from build123d import *

# Parameters (mm, degrees)
SKETCH1_R           = 2.5
SKETCH1_R_2         = 2
BOSS_EXTRUDE1_DEPTH = 5
SKETCH2_R           = 2.85
CUT_EXTRUDE1_DEPTH  = 8
CHAMFER1_SIZE       = 0.5
SKETCH3_W           = 22
SKETCH3_H           = 55
CUT_EXTRUDE2_DEPTH  = 5


with BuildPart() as part:
    # Sketch1 → Boss-Extrude1 (new, symmetric)
    with BuildSketch(Plane(origin=(0, 0, 0), x_dir=(1, 0, 0), z_dir=(0, 1, 0))):
        Polygon((27.5, 27.5), (-27.5, 27.5), (-27.5, -27.5), (27.5, -27.5), (27.5, -11), (24.5, -11), (24.5, 11), (27.5, 11), align=None)
        with Locations(Location((-14.4, -17.5, 0), (0, 0, 270))):
            Circle(SKETCH1_R, mode=Mode.SUBTRACT)
        with Locations(Location((14.4, -17.5, 0), (0, 0, 270))):
            Circle(SKETCH1_R, mode=Mode.SUBTRACT)
        with Locations(Location((14.4, -7.5, 0), (0, 0, 270))):
            Circle(SKETCH1_R_2, mode=Mode.SUBTRACT)
        with Locations(Location((-14.4, 17.5, 0), (0, 0, 270))):
            Circle(SKETCH1_R, mode=Mode.SUBTRACT)
        with Locations(Location((14.4, 7.5, 0), (0, 0, 270))):
            Circle(SKETCH1_R_2, mode=Mode.SUBTRACT)
        with Locations(Location((14.4, 17.5, 0), (0, 0, 270))):
            Circle(SKETCH1_R, mode=Mode.SUBTRACT)
    extrude(amount=BOSS_EXTRUDE1_DEPTH, both=True)

    # Sketch2 → Cut-Extrude1 (cut)
    with BuildSketch(Plane.XY.offset(27.5)):
        with Locations((-22, 0)):
            Circle(SKETCH2_R)
        with Locations(Location((22, 0, 0), (0, 0, 180))):
            Circle(SKETCH2_R)
    cut_extrude1 = extrude(amount=-CUT_EXTRUDE1_DEPTH, mode=Mode.SUBTRACT)

    # Mirror1: Cut-Extrude1 across plane
    add(cut_extrude1.mirror(Plane.XY), mode=Mode.SUBTRACT)

    # Chamfer1
    chamfer1_edges = [part.edges().sort_by_distance(p)[0] for p in [
        (14.4, 5, 5.5),
        (14.4, 5, -9.5),
        (-24.85, 0, 27.5),
        (24.85, 0, 27.5),
        (-24.85, 0, -27.5),
        (24.85, 0, -27.5),
    ]]
    chamfer(chamfer1_edges, length=CHAMFER1_SIZE)

    # Sketch3 → Cut-Extrude2 (cut)
    with BuildSketch(Plane(origin=(0, 5, 0), x_dir=(1, 0, 0), z_dir=(0, 1, 0))):
        Rectangle(SKETCH3_W, SKETCH3_H)
    extrude(amount=-CUT_EXTRUDE2_DEPTH, mode=Mode.SUBTRACT)


solid = part.part
Here's how the part is built. I have some questions about the finished solid (model axes, mm). A direction names the side the tool comes from. Coordinates: 2 decimals unless noted, no trailing zeros. Order: outer loops, then holes, each group sorted by start corner. A loop starts at its lowest first (then second) coordinate and runs counter-clockwise, first axis right, second up. Notation, with made-up numbers: (-10.75, 34) -> (3.25, 34) arc R33 ccw to (3.25, 68) -> close; hole circle Ø3 at (-19, -28). An arc over 180 degrees is marked (long way). Answer in a Markdown table with one row per item.
(1) I want a section at D-D on x = -14.4. List the corners of the cut face in (y, z) for me.
Answer key:
| item | result |
|---|---|
| outline | (-5, -27.5) -> (5, -27.5) -> (5, -20) -> (-5, -20) -> close; (-5, -15) -> (5, -15) -> (5, 15) -> (-5, 15) -> close; (-5, 20) -> (5, 20) -> (5, 27.5) -> (-5, 27.5) -> close |
(2) Will these pins go through, and if not, where does the flat tip stop? pin 1 Ø1.5 at (y, z) = (2, 3) entering from +X; pin 2 Ø4.5 at (x, y) = (22, 0) entering from +Z; pin 3 Ø3 at (x, z) = (14.4, -17.5) entering from -Y; pin 4 Ø5 at (x, z) = (-2.5, -11) entering from +Y.
Answer key:
| item | result |
|---|---|
| pin 1 | x = 24.5 |
| pin 2 | z = 19.5 |
| pin 3 | through |
| pin 4 | y = 0 |
(3) Please list where these lines run through material, in increasing order: probe 1 along X at (y, z) = (-2, -17.5); probe 2 along X at (y, z) = (-4, 16); probe 3 along X at (y, z) = (1.75, -18.5).
Answer key:
| item | result |
|---|---|
| probe 1 | -27.5 to -16.9, -11.9 to 11.9, 16.9 to 27.5 |
| probe 2 | -27.5 to -16.4, -12.4 to 12.4, 16.4 to 27.5 |
| probe 3 | -27.5 to -16.69, -12.11 to -11, 11 to 12.11, 16.69 to 27.5 |
(4) I want a section at A-A on x = 14.4. List the corners of the cut face in (y, z) for me.
Answer key:
| item | result |
|---|---|
| outline | (-5, -27.5) -> (5, -27.5) -> (5, -20) -> (-5, -20) -> close; (-5, -15) -> (5, -15) -> (5, -10) -> (4.5, -9.5) -> (-5, -9.5) -> close; (-5, -5.5) -> (4.5, -5.5) -> (5, -5) -> (5, 5) -> (4.5, 5.5) -> (-5, 5.5) -> close; (-5, 9.5) -> (4.5, 9.5) -> (5, 10) -> (5, 15) -> (-5, 15) -> close; (-5, 20) -> (5, 20) -> (5, 27.5) -> (-5, 27.5) -> close |
(5) I want a section at C-C on z = 7.5. List the corners of the cut face in (x, y) for me.
Answer key:
| item | result |
|---|---|
| outline | (-27.5, -5) -> (12.4, -5) -> (12.4, 4.5) -> (11.9, 5) -> (11, 5) -> (11, 0) -> (-11, 0) -> (-11, 5) -> (-27.5, 5) -> close; (16.4, -5) -> (24.5, -5) -> (24.5, 5) -> (16.9, 5) -> (16.4, 4.5) -> close |
(6) Thinking about a two-plate mould opening in Y: for faces 4 (the face through (22.62, 2.78, 23.3)), 5 (the face through (14.5, -0.1, 15)), 6 (the face through (0, 0, 0)), which applies, +Y half, -Y half, draft (parallel to the pull), parting line (faces both ways), or undercut?
Answer key:
| item | result |
|---|---|
| face 4 | undercut |
| face 5 | draft |
| face 6 | +Y half |
(7) I want a section at B-B on z = 17.5. List the corners of the cut face in (x, y) for me, then the cut area to 3 significant figures.
Answer key:
| item | result |
|---|---|
| outline | (-27.5, -5) -> (-16.9, -5) -> (-16.9, 5) -> (-27.5, 5) -> close; (-11.9, -5) -> (11.9, -5) -> (11.9, 5) -> (11, 5) -> (11, 0) -> (-11, 0) -> (-11, 5) -> (-11.9, 5) -> close; (16.9, -5) -> (27.5, -5) -> (27.5, 5) -> (16.9, 5) -> close |
| area | 340 mm^2 |
(8) On a 3-axis mill with a long thin cutter (end or side, diameter ignored), from which of +Z, -Z, +X, -X, +Y, -Y can I reach the whole of each face in a straight line? I mean faces 1 (the face through (24.5, 0, 0)), 2 (the face through (22, 0, -19.5)), 3 (the face through (-22, 0, 19.5)). Say none if no direction works.
Answer key:
| item | result |
|---|---|
| face 1 | +X, +Y, -Y |
| face 2 | -Z |
| face 3 | +Z |
